```python
from build123d import *

# Parameters (mm, degrees)
SKETCH1_W                 = 393.7
SKETCH1_H                 = 229.108
BASE_FLANGE1_DEPTH        = 1.5875
MITER_START               = -196.85
MITER_FLANGE1_DEPTH       = 393.7
MITER_FLANGE1_2_DEPTH     = 393.7
F_8_CLEARANCE_HOLE1_D     = 4.3053
F_8_CLEARANCE_HOLE1_DEPTH = 1.5875
FILLET1_R                 = 2.54


# Read off the part's stored shape, not the designer's step: Miter Flange1
# Sheet-metal steps are written as plain solids
with BuildPart() as part:
    # Sketch1 → Base-Flange1 (new body)
    with BuildSketch(Plane(origin=(0, 0, 0), x_dir=(1, 0, 0), z_dir=(0, 1, 0))):
        Rectangle(SKETCH1_W, SKETCH1_H)
    extrude(amount=-BASE_FLANGE1_DEPTH)

    # Miter Flange1 outline → Miter Flange1 (cut)
    with BuildSketch(Plane.YZ.offset(MITER_START)):
        with BuildLine():
            Line((-1.5875, -114.554), (-1.467682479, -114.554))
            ThreePointArc((-1.467682479, -114.554), (-1.557350056, -114.190540657), (-1.5875, -113.8174))
            Line((-1.5875, -113.8174), (-1.5875, -114.554))
        make_face()
    miter_flange1 = extrude(amount=MITER_FLANGE1_DEPTH, mode=Mode.SUBTRACT)

    # Miter Flange1 2 outline → Miter Flange1 2 (add)
    with BuildSketch(Plane.YZ.offset(MITER_START)):
        with BuildLine():
            Line((39.6875, -113.8174), (39.6875, -92.329))
            Line((39.6875, -92.329), (38.1, -92.329))
            Line((38.1, -92.329), (38.1, -113.8174))
            ThreePointArc((38.1, -113.8174), (37.884254855, -114.338254855), (37.3634, -114.554))
            Line((37.3634, -114.554), (0.7366, -114.554))
            ThreePointArc((0.7366, -114.554), (0.215745145, -114.338254855), (0, -113.8174))
            Line((0, -113.8174), (0, -114.554))
            Line((0, -114.554), (-1.467682479, -114.554))
            ThreePointArc((-1.467682479, -114.554), (-0.621617352, -115.703317929), (0.7366, -116.1415))
            Line((0.7366, -116.1415), (37.3634, -116.1415))
            ThreePointArc((37.3634, -116.1415), (39.00678687, -115.46078687), (39.6875, -113.8174))
        make_face()
    miter_flange1_2 = extrude(amount=MITER_FLANGE1_2_DEPTH)

    # Mirror1: Miter Flange1, Miter Flange1 2 across plane
    add(miter_flange1.mirror(Plane.XY), mode=Mode.SUBTRACT)
    add(miter_flange1_2.mirror(Plane.XY))

    # #8 Clearance Hole1
    with Locations(Plane(origin=(0, 39.6875, 0), x_dir=(1, 0, 0), z_dir=(0, 1, 0))):
        with Locations((166.207772673, -109.057772673), (46.99, -109.057772673), (-72.39, -109.057772673), (-191.607772673, -109.057772673), (-191.607772673, 109.057772673), (-72.39, 109.057772673), (46.99, 109.057772673), (166.207772673, 109.057772673)):
            Hole(F_8_CLEARANCE_HOLE1_D / 2, depth=F_8_CLEARANCE_HOLE1_DEPTH)

    # Fillet1
    fillet1_edges = [part.edges().sort_by_distance(p)[0] for p in [
        (-196.85, 38.89375, -92.329),
        (196.85, 38.89375, -92.329),
        (-196.85, 38.89375, 92.329),
        (196.85, 38.89375, 92.329),
    ]]
    fillet(fillet1_edges, radius=FILLET1_R)


solid = part.part
```
Design review of the part built by this model. Coordinates are the model's own, in mm. A direction names the side the tool comes from. Coordinates: 2 decimals unless noted, no trailing zeros. Write each loop counter-clockwise with the first axis right and the second up, starting at its lowest first coordinate (ties: lowest second). Pieces come first, ordered by that corner, then holes.
1) Machinability: for faces 1 (the flat face through (-3, 38.1, 103)), 2 (the flat face through (-196.85, -1, -1)), which of the approach directions +Z, -Z, +X, -X, +Y, -Y give a long, thin tool a straight path to every point of the face, cutting with its end or side? Answer none if there is none.
2) Insertion check: pin 1 (0.8 mm diameter, centred on x = 34, y = 39, fed in from +Z); pin 2 (12 mm diameter, centred on x = -24, z = 53, fed in from +Y); pin 3 (1.3 mm diameter, centred on x = -48.5, y = 39, fed in from -Z). Each pin has a flat end and moves straight along its axis. Give the tip position at first contact, or say it passes through.
3) Add section B-B (x = 90.5). Write out the cut boundary in (y, z).
4) Mouldability with a two-part tool opening along Y and no side actions: class faces 3 (the flat face through (-3, 19, -114.554)), 4 (the flat face through (196.85, -1, -1)), 5 (the flat face through (-3, 39.688, 103)), 6 (the flat face through (-3, 19, 114.554)) as +Y half, -Y half, draft (parallel to the pull), parting line (faces both ways), or undercut.
5) Add section C-C (z = -50). Write out the cut boundary in (x, y).
6) To check wall thickness, follow L1, parallel to Z at x = -140.5, y = 7; L2, parallel to Y at x = -74.5, z = 101; L3, parallel to Z at x = -72.39, y = 38.65. State the ranges of each line that lie inside material, in increasing order.
7) Add section A-A (y = 19). Write out the cut boundary in (x, z).
Check result:
1. face 1: +X, -X
1. face 2: +Z, -Z, -X, +Y, -Y
2. pin 1: stops at z = 115.79
2. pin 2: stops at y = 0
2. pin 3: stops at z = -115.92
3. outline: (-1.59, -113.82) arc R2.32 ccw to (0.74, -116.14) - (37.36, -116.14) arc R2.32 ccw to (39.69, -113.82) - (39.69, -92.33) - (38.1, -92.33) - (38.1, -113.82) arc R0.74 cw to (37.36, -114.55) - (0.74, -114.55) arc R0.74 cw to (0, -113.82) - (0, 113.82) arc R0.74 cw to (0.74, 114.55) - (37.36, 114.55) arc R0.74 cw to (38.1, 113.82) - (38.1, 92.33) - (39.69, 92.33) - (39.69, 113.82) arc R2.32 ccw to (37.36, 116.14) - (0.74, 116.14) arc R2.32 ccw to (-1.59, 113.82) - close
4. face 3: undercut
4. face 4: draft
4. face 5: +Y half
4. face 6: undercut
5. outline: (-196.85, -1.59) - (196.85, -1.59) - (196.85, 0) - (-196.85, 0) - close
6. L1: z = -116.14 to -114.55, 114.55 to 116.14
6. L2: y = -1.59 to 0, 38.1 to 39.69
6. L3: z = -115.75 to -111.21, -106.91 to -92.33, 92.33 to 106.91, 111.21 to 115.75
7. outline: (-196.85, -116.14) - (196.85, -116.14) - (196.85, -114.55) - (-196.85, -114.55) - close; (-196.85, 114.55) - (196.85, 114.55) - (196.85, 116.14) - (-196.85, 116.14) - close
